Check sheet for the drawn part. Datum: minimum x, y, z corner. Units: mm. Round coordinates to 2 decimals unless told otherwise and drop trailing zeros. Write each loop counter-clockwise with the first axis right and the second up, starting at its lowest first coordinate (ties: lowest second). Pieces come first, ordered by that corner, then holes. Notation, with made-up numbers: M 86,17 L 115,17 A20 cw 115,41 Z; hole C 40,-24.75 d9. An arc over 180 degrees is marked long. One line per item, written item: value. Start each with the question number.
1. Section check A-A (x = 30). Record the boundary of the cut face in (y, z), and give its area (3 significant figures).
2. Scan lines: probe 1 along X at (y, z) = (18, 0.95); probe 2 along Y at (x, z) = (21, 1.15); probe 3 along X at (y, z) = (28.5, 1.5). Record each from-to range of solid material in increasing order. Write a range as [from, to].
3. Section check D-D (y = 2). Record the boundary of the cut face in (x, z), and give its area (3 significant figures).
4. Release check for a two-part mould opening along Z. For the marked faces 1 and 2 record: pulls with the +Z half, pulls with the -Z half, needs draft (parallel to the pull), parting line crosses it, or undercut.
5. Section check C-C (z = 1.3). Record the boundary of the cut face in (x, y), and give its area (3 significant figures).
6. Section check B-B (y = 19). Record the boundary of the cut face in (x, z), and give its area (3 significant figures).
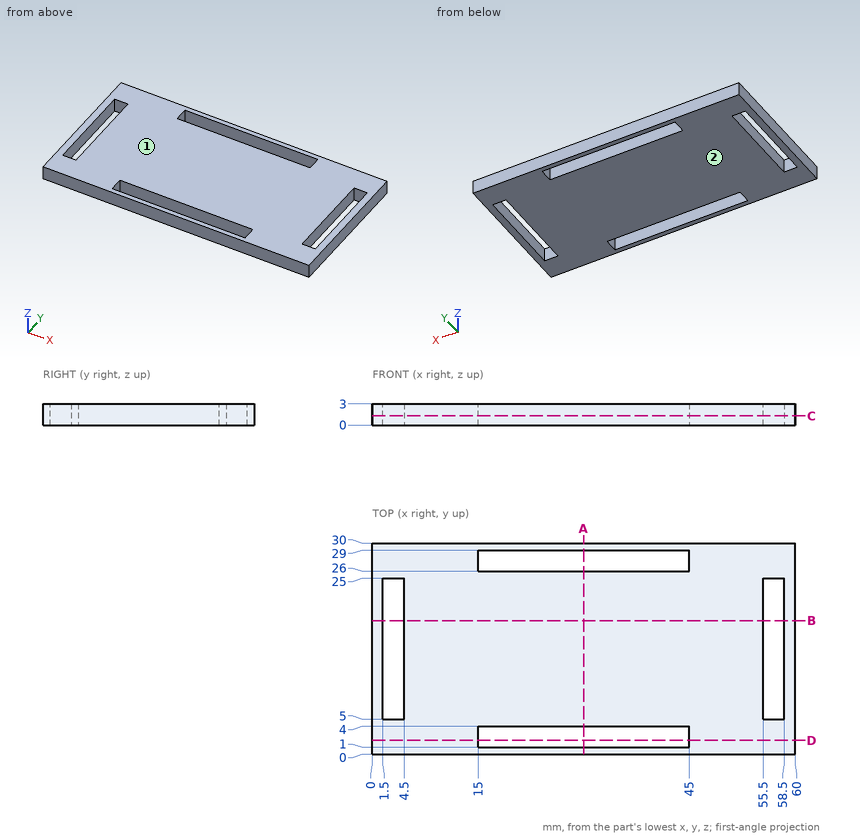
Result sheet:
1. outline: M 0,0 L 1,0 L 1,3 L 0,3 Z; M 4,0 L 26,0 L 26,3 L 4,3 Z; M 29,0 L 30,0 L 30,3 L 29,3 Z
1. area: 72.0 mm2
2. probe 1: x = [0, 1.5], [4.5, 55.5], [58.5, 60]
2. probe 2: y = [0, 1], [4, 26], [29, 30]
2. probe 3: x = [0, 15], [45, 60]
3. outline: M 0,0 L 15,0 L 15,3 L 0,3 Z; M 45,0 L 60,0 L 60,3 L 45,3 Z
3. area: 90.0 mm2
4. face 1: pulls with the +Z half
4. face 2: pulls with the -Z half
5. outline: M 0,0 L 60,0 L 60,30 L 0,30 Z; hole M 1.5,5 L 4.5,5 L 4.5,25 L 1.5,25 Z; hole M 15,1 L 45,1 L 45,4 L 15,4 Z; hole M 15,26 L 45,26 L 45,29 L 15,29 Z; hole M 55.5,5 L 58.5,5 L 58.5,25 L 55.5,25 Z
5. area: 1,500 mm2
6. outline: M 0,0 L 1.5,0 L 1.5,3 L 0,3 Z; M 4.5,0 L 55.5,0 L 55.5,3 L 4.5,3 Z; M 58.5,0 L 60,0 L 60,3 L 58.5,3 Z
6. area: 162 mm2
